Autodesk Inventor part; units mm, degrees
ref_plane "YZ Plane" through (0, 0, 0) normal (1, 0, 0) x (0, 1, 0)
ref_plane "XZ Plane" through (0, 0, 0) normal (0, 1, 0) x (-1, 0, 0)
ref_plane "XY Plane" through (0, 0, 0) normal (0, 0, 1) x (1, 0, 0)
sketch "Sketch1" plane through (0, 0, 0) normal (0, 0, 1) x (1, 0, 0)
  line L0 (131.3749, -73.5016) -> (131.3749, -71.6344)
  arc A0 (131.3749, -71.6344) -> (89.8052, -1.2952) centre (51.0805, -71.6344) ccw
  arc A1 (89.8052, -1.2952) -> (84.0169, -0.1805) centre (84.7113, -12.1604) ccw
  line L1 (84.0169, -0.1805) -> (0.0993, 0.1926)
  line L2 (0.0993, 0.1926) -> (-0.2975, -89.0508)
  arc A2 (-0.2975, -89.0508) -> (7.9081, -98.4818) centre (9.6942, -88.6426) ccw
  circle A3 centre (120.9184, -82.9714) radius 3.3
  arc A4 (145.7873, -114.287) -> (148.0883, -110.4202) centre (146.9636, -112.3689) ccw
  arc A5 (145.7873, -124.287) -> (148.0882, -120.4202) centre (146.9636, -122.3689) ccw
  circle A6 centre (22.531, -40.6102) radius 2.8
  circle A7 centre (28.6758, -122.3689) radius 2.25
  circle A8 centre (28.6758, -112.3689) radius 2.25
  circle A9 centre (10, -88.6441) radius 3.3
  arc A10 (32.2446, -127.2916) -> (33.2446, -128.2916) centre (33.2446, -127.2916) ccw
  line L3 (32.2446, -127.2916) -> (32.2446, -107.4916)
  arc A11 (33.2446, -106.4916) -> (32.2446, -107.4916) centre (33.2446, -107.4916) ccw
  arc A12 (142.8483, -107.4916) -> (141.8483, -106.4916) centre (141.8483, -107.4916) ccw
  line L4 (142.8483, -107.4916) -> (142.8483, -127.2916)
  arc A13 (141.8483, -128.2916) -> (142.8483, -127.2916) centre (141.8483, -127.2916) ccw
  circle A14 centre (146.9636, -112.3689) radius 2.25
  circle A15 centre (146.9636, -122.3689) radius 2.25
  circle A16 centre (43.0964, -117.3689) radius 6
  circle A17 centre (131.9964, -117.3688) radius 6
  circle A18 centre (78.1699, -22.3386) radius 3.25
  circle A19 centre (78.1699, -22.3386) radius 6
  arc A20 (131.9964, -138.3688) -> (144.7874, -100.7138) centre (131.9964, -117.3688) ccw
  arc A21 (22.0858, -117.7084) -> (7.9081, -98.4818) centre (1.5094, -118.0409) ccw
  arc A22 (131.3749, -73.5016) -> (144.7874, -100.7138) centre (165.6862, -73.5016) ccw
  arc A23 (22.0858, -117.7084) -> (42.3476, -138.3689) centre (43.0964, -117.3689) ccw
  arc A24 (109.9151, -129.4423) -> (65.1778, -129.4423) centre (87.5464, -138.1396) ccw
  line L5 (42.3476, -138.3689) -> (52.1294, -138.3689)
  line L6 (122.9635, -138.3688) -> (131.9964, -138.3688)
  arc A25 (52.1294, -138.3689) -> (65.1778, -129.4423) centre (52.1294, -124.3689) ccw
  arc A26 (109.9151, -129.4423) -> (122.9635, -138.3688) centre (122.9635, -124.3688) ccw
  circle A27 centre (43.0964, -117.3689) radius 4.6
  line L7 (1.9461, -54.0938) -> (33.2975, -54.0938) construction
  line L8 (33.2975, -54.0938) -> (33.2975, -61.1615) construction
  line L9 (33.2975, -61.1615) -> (1.9461, -61.1615) construction
  line L10 (1.9461, -61.1615) -> (1.9461, -54.0938) construction
  circle A28 centre (79.294, -41.6199) radius 2.8
  circle A29 centre (78.1699, -22.3386) radius 6
  circle A30 centre (22.531, -40.6102) radius 2.8
  circle A31 centre (22.6705, -8.6105) radius 2.8
  circle A32 centre (22.6705, -8.6105) radius 2.8
  circle A33 centre (120.9184, -82.9714) radius 3.3
  line L11 (2.1801, -54.1888) -> (3.0075, -54.1888)
  spline S0 degree 2 poles (3.0075, -54.1888) (3.8349, -54.1888) (4.4216, -54.3176) (4.7912, -54.8433) (4.7912, -55.4164) knots 0 0 0 1 2 3 3 3
  spline S1 degree 2 poles (4.7912, -55.4164) (4.7912, -55.942) (4.5301, -56.3048) (4.1469, -56.3421) knots 0 0 0 1 2 2 2
  spline S2 degree 2 poles (4.1469, -56.3421) (4.4928, -56.4269) (4.7336, -56.7152) (4.7912, -56.9559) (4.7912, -57.5019) knots 0 0 0 1 2 3 3 3
  line L12 (4.7912, -57.5019) -> (4.7912, -58.6888)
  line L13 (4.7912, -58.6888) -> (3.7027, -58.6888)
  line L14 (3.7027, -58.6888) -> (3.7027, -57.1933)
  spline S3 degree 2 poles (3.7027, -57.1933) (3.7027, -56.8338) (3.5908, -56.6609) (3.35, -56.6609) knots 0 0 0 1 2 2 2
  line L15 (3.35, -56.6609) -> (3.35, -58.6888)
  line L16 (3.35, -58.6888) -> (2.1801, -58.6888)
  line L17 (2.1801, -58.6888) -> (2.1801, -54.1888)
  line L18 (3.35, -54.9586) -> (3.35, -55.9589)
  spline S4 degree 2 poles (3.35, -55.9589) (3.5467, -55.9589) (3.7027, -55.8504) (3.7027, -55.552) knots 0 0 0 1 2 2 2
  line L19 (3.7027, -55.552) -> (3.7027, -55.3045)
  spline S5 degree 2 poles (3.7027, -55.3045) (3.7027, -55.0908) (3.5501, -54.9586) (3.35, -54.9586) knots 0 0 0 1 2 2 2
  line L20 (6.5851, -56.454) -> (6.5851, -57.2306)
  line L21 (6.5851, -57.2306) -> (5.1134, -57.2306)
  line L22 (5.1134, -57.2306) -> (5.1134, -56.454)
  line L23 (5.1134, -56.454) -> (6.5851, -56.454)
  spline S6 degree 2 poles (9.593, -56.8237) (9.593, -57.5019) (9.5286, -58.0648) (9.1929, -58.5328) (8.6198, -58.7837) (8.24, -58.7837) knots 0 0 0 1 2 3 4 4 4
  spline S7 degree 2 poles (8.24, -58.7837) (7.8771, -58.7837) (7.304, -58.5464) (6.9548, -58.075) (6.8869, -57.5189) (6.8869, -56.8237) knots 0 0 0 1 2 3 4 4 4
  line L24 (6.8869, -56.8237) -> (6.8869, -56.0539)
  spline S8 degree 2 poles (6.8869, -56.0539) (6.8869, -55.3757) (6.9514, -54.8127) (7.2871, -54.3448) (7.8602, -54.0938) (8.24, -54.0938) knots 0 0 0 1 2 3 4 4 4
  spline S9 degree 2 poles (8.24, -54.0938) (8.6028, -54.0938) (9.1759, -54.3312) (9.5252, -54.8026) (9.593, -55.3587) (9.593, -56.0539) knots 0 0 0 1 2 3 4 4 4
  line L25 (9.593, -56.0539) -> (9.593, -56.8237)
  spline S10 degree 2 poles (8.4231, -55.3452) (8.4231, -55.0332) (8.3553, -54.8568) (8.2468, -54.8568) knots 0 0 0 1 2 2 2
  spline S11 degree 2 poles (8.2468, -54.8568) (8.1552, -54.8568) (8.0569, -54.9993) (8.0569, -55.3452) knots 0 0 0 1 2 2 2
  line L26 (8.0569, -55.3452) -> (8.0569, -57.4442)
  spline S12 degree 2 poles (8.0569, -57.4442) (8.0569, -57.8376) (8.1213, -58.0207) (8.2366, -58.0207) knots 0 0 0 1 2 2 2
  spline S13 degree 2 poles (8.2366, -58.0207) (8.3553, -58.0207) (8.4231, -57.8105) (8.4231, -57.4137) knots 0 0 0 1 2 2 2
  line L27 (8.4231, -57.4137) -> (8.4231, -55.3452)
  line L28 (12.6891, -54.1888) -> (12.6891, -57.1967)
  spline S14 degree 2 poles (12.6891, -57.1967) (12.6891, -57.7088) (12.6213, -58.1225) (12.2958, -58.5599) (11.76, -58.7837) (11.3937, -58.7837) knots 0 0 0 1 2 3 4 4 4
  spline S15 degree 2 poles (11.3937, -58.7837) (10.9902, -58.7837) (10.3764, -58.5158) (10.0678, -58.0886) (10.0135, -57.6138) (10.0135, -56.8508) knots 0 0 0 1 2 3 4 4 4
  line L29 (10.0135, -56.8508) -> (10.0135, -54.1888)
  line L30 (10.0135, -54.1888) -> (11.1835, -54.1888)
  line L31 (11.1835, -54.1888) -> (11.1835, -57.5629)
  spline S16 degree 2 poles (11.1835, -57.5629) (11.1835, -57.858) (11.2479, -58.0207) (11.3429, -58.0207) knots 0 0 0 1 2 2 2
  spline S17 degree 2 poles (11.3429, -58.0207) (11.4548, -58.0207) (11.5192, -57.841) (11.5192, -57.5053) knots 0 0 0 1 2 2 2
  line L32 (11.5192, -57.5053) -> (11.5192, -54.1888)
  line L33 (11.5192, -54.1888) -> (12.6891, -54.1888)
  line L34 (15.5004, -54.1888) -> (15.5004, -55.0908)
  line L35 (15.5004, -55.0908) -> (14.8052, -55.0908)
  line L36 (14.8052, -55.0908) -> (14.8052, -58.6888)
  line L37 (14.8052, -58.6888) -> (13.6352, -58.6888)
  line L38 (13.6352, -58.6888) -> (13.6352, -55.0908)
  line L39 (13.6352, -55.0908) -> (12.9435, -55.0908)
  line L40 (12.9435, -55.0908) -> (12.9435, -54.1888)
  line L41 (12.9435, -54.1888) -> (15.5004, -54.1888)
  point P0 (0, 0)
  point P1 (58.8546, -117.3689)
  point P2 (63.5475, -138.3689)
  point P3 (111.5453, -138.3689)
  dimension "d6" = 10
  dimension "d7" = 12
  dimension "d10" = 88.9
  dimension "d11" = 42
  dimension "d13" = 10.8518
  dimension "d14" = 10.8518
  dimension "d16" = 4.1153
  dimension "d17" = 4.1153
  dimension "d18" = 48
  dimension "d19" = 14
  dimension "d20" = 44.45
  dimension "d23" = 5.6
  dimension "d25" = 56.763
  dimension "d26" = 19.314
  dimension "d27" = 78.17
extrude "Extrusion1" add sketch "Sketch1" along normal blind 4.1153 contours A22 A20 L6 A26 A24 A25 L5 A23 A21 A2 L2 L1 A1 A0 L0 | A14 A4 | A15 A5 | A7 | A8 | A9 | L11 S0 S1 S2 L12 L13 L14 S3 L15 L16 L17 | S5 L19 S4 L18 | L20 L21 L22 L23 | S6 S7 L24 S8 S9 L25 | L27 S13 S12 L26 S11 S10 | L28 S14 S15 L29 L30 L31 S16 S17 L32 L33 | L34 L35 L36 L37 L38 L39 L40 L41
extrude "Extrusion2" cut sketch "Sketch1" against normal blind 1 from surface at 4.1153 contours L11 S0 S1 S2 L12 L13 L14 S3 L15 L16 L17 | L20 L21 L22 L23 | S6 S7 L24 S8 S9 L25 | L28 S14 S15 L29 L30 L31 S16 S17 L32 L33 | L34 L35 L36 L37 L38 L39 L40 L41
equation "\"d14\" = d13"
equation "\"d16\" = d15"
equation "\"d17\" = d15"
equation "\"d20\" = 0.5 * d10"
equation "\"d0\" = d16"
properties part number "Intake Sides V6ipt" material "Polycarbonate, Clear"
Input: part model. Units: mm. Frame: model coordinates. A direction names the side the tool comes from. Give positions to 0.01 mm unless a question says otherwise; leave off trailing zeros. Order: outer loops, then holes, each group sorted by start corner. A loop starts at its lowest first (then second) coordinate and runs counter-clockwise, first axis right, second up. Notation, with made-up numbers: M -5,0 L 2,0 A12 cw 2,15 Z; hole C 12,28.5 d6. An arc over 180 degrees is marked long. Answer as a JSON object with one key per item and string values.
1. Cut plane A-A, the plane z = 1. Output: boundary loops of the cut face in (x, y), and give its area (3 significant figures).
Result sheet:
{"outline": "M -0.3,-89.05 A10 ccw 7.91,-98.48 A20.58 cw 22.09,-117.71 A21.01 ccw 42.35,-138.37 L 52.13,-138.37 A14 ccw 65.18,-129.44 A24 cw 109.92,-129.44 A14 ccw 122.96,-138.37 L 132,-138.37 A21 ccw 144.79,-100.71 A34.31 cw 131.37,-73.5 L 131.37,-71.63 A80.29 ccw 89.81,-1.3 A12 ccw 84.02,-0.18 L 0.1,0.19 Z; hole C 22.53,-40.61 d5.6; hole C 22.67,-8.61 d5.6; hole C 43.1,-117.37 d12; hole C 78.17,-22.34 d12; hole C 79.29,-41.62 d5.6; hole C 120.92,-82.97 d6.6; hole C 132,-117.37 d12", "area": "15,700 mm²"}
2. Ray query, line 1 (Y direction, x = 119, z = 2.9); line 2 (X direction, y = -132, z = 3.4); line 3 (X direction, y = -124, z = 3). Return the intervals inside material, ascending. Write a range as [from, to].
Result sheet:
{"line 1": "[-137.8, -85.66], [-80.29, -28.81]", "line 2": "[28.01, 63.87], [111.23, 147.06]", "line 3": "[23.16, 68.15], [106.94, 151.92]"}
3. Cut plane C-C, the plane y = -63. Output: boundary loops of the cut face in (x, z), and give its area (3 significant figures).
Result sheet:
{"outline": "M -0.18,0 L 130.91,0 L 130.91,4.12 L -0.18,4.12 Z", "area": "539 mm²"}
4. Pull-direction query (X, two-part tool) for faces 3 (the cylindrical face through (115.16, -135.99, 2.03)), 4 (the flat face through (47, -138.369, 2)), 5 (the cylindrical face through (17.966, -105.684, 2.029)); classes: +X half, -X half, draft (parallel to the pull), parting line (faces both ways), or undercut.
Result sheet:
{"face 3": "undercut", "face 4": "draft", "face 5": "-X half"}
5. Cut plane B-B, the plane x = 115.5. Output: boundary loops of the cut face in (y, z), and give its area (3 significant figures).
Result sheet:
{"outline": "M -136.21,0 L -23.7,0 L -23.7,4.12 L -136.21,4.12 Z", "area": "463 mm²"}
6. Reachability of faces 1 (the flat face through (75, -68, 4.115)), 2 (the cylindrical face through (60.13, -135.86, 2.03)) from +Z, -Z, +X, -X, +Y, -Y: full face, straight path, thin tool, end or side. Return the list, or none.
Result sheet:
{"face 1": "+Z, +X, -X, +Y, -Y", "face 2": "+Z, -Z, -Y"}
7. First-contact query: P1, Ø1.1, axis at y = -56, z = 4, coming from the +X side; P2, Ø0.5, axis at x = 4.5, z = 3.5, coming from the +Y side; P3, Ø0.9, axis at y = -56.5, z = 3.5, coming from the -X side; P4, Ø5, axis at x = 79.29, y = -41.62, coming from the +Z side. Flat tips, straight axial feed; report the tip coordinate or a pass-through.
Result sheet:
{"P1": "x = 129.95", "P2": "y = 0.17", "P3": "x = -0.15", "P4": "through"}
